Could you check a few things on this model? Use its own coordinates, in mm. A direction names the side the tool comes from. Coordinates: 2 decimals unless noted, no trailing zeros. Order: outer loops, then holes, each group sorted by start corner. A loop starts at its lowest first (then second) coordinate and runs counter-clockwise, first axis right, second up.
```python
from build123d import *

# Parameters (mm, degrees)
ESQUISSE1_W                                   = 30
ESQUISSE1_H                                   = 30
ESQUISSE1_R                                   = 12.5
BOSS_EXTRU_1_DEPTH                            = 6
ESQUISSE3_R                                   = 13
ENL_V_MAT_EXTRU_1_DEPTH                       = 5
TROU_POUR_TARAUDAGE_POUR_TROU_TARAUD_M3_D     = 2.5
TROU_POUR_TARAUDAGE_POUR_TROU_TARAUD_M3_DEPTH = 6
TROU_POUR_TARAUDAGE_POUR_TROU_TARAUD_M3_TIP   = 0.751075774
TROU_POUR_TARAUDAGE_POUR_TROU_TARAUD_2_D      = 2.5
TROU_POUR_TARAUDAGE_POUR_TROU_TARAUD_2_DEPTH  = 6
TROU_POUR_TARAUDAGE_POUR_TROU_TARAUD_2_TIP    = 0.751075774


with BuildPart() as part:
    # Esquisse1 → Boss.-Extru.1 (new body)
    with BuildSketch(Plane.XY):
        with Locations((15, 15)):
            Rectangle(ESQUISSE1_W, ESQUISSE1_H)
        with Locations((15, 15)):
            Circle(ESQUISSE1_R, mode=Mode.SUBTRACT)
    extrude(amount=BOSS_EXTRU_1_DEPTH)

    # Esquisse3 → Enlèv. mat.-Extru.1 (cut)
    with BuildSketch(Plane.XY.offset(6)):
        with Locations((15, 15)):
            Circle(ESQUISSE3_R)
    extrude(amount=-ENL_V_MAT_EXTRU_1_DEPTH, mode=Mode.SUBTRACT)

    # Trou pour taraudage pour trou taraud_ M3
    with Locations(Plane(origin=(0, 30, 0), x_dir=(1, 0, 0), z_dir=(0, 1, 0))):
        with Locations((2, -3), (28, -3)):
            Hole(TROU_POUR_TARAUDAGE_POUR_TROU_TARAUD_M3_D / 2, depth=TROU_POUR_TARAUDAGE_POUR_TROU_TARAUD_M3_DEPTH)
            with Locations((0, 0, -(TROU_POUR_TARAUDAGE_POUR_TROU_TARAUD_M3_DEPTH + TROU_POUR_TARAUDAGE_POUR_TROU_TARAUD_M3_TIP / 2))):  # 118° drill point
                Cone(0, TROU_POUR_TARAUDAGE_POUR_TROU_TARAUD_M3_D / 2, TROU_POUR_TARAUDAGE_POUR_TROU_TARAUD_M3_TIP, mode=Mode.SUBTRACT)

    # Trou pour taraudage pour trou taraud 2
    with Locations(Plane(origin=(0, 0, 0), x_dir=(-1, 0, 0), z_dir=(0, -1, 0))):
        with Locations((-2, -3), (-28, -3)):
            Hole(TROU_POUR_TARAUDAGE_POUR_TROU_TARAUD_2_D / 2, depth=TROU_POUR_TARAUDAGE_POUR_TROU_TARAUD_2_DEPTH)
            with Locations((0, 0, -(TROU_POUR_TARAUDAGE_POUR_TROU_TARAUD_2_DEPTH + TROU_POUR_TARAUDAGE_POUR_TROU_TARAUD_2_TIP / 2))):  # 118° drill point
                Cone(0, TROU_POUR_TARAUDAGE_POUR_TROU_TARAUD_2_D / 2, TROU_POUR_TARAUDAGE_POUR_TROU_TARAUD_2_TIP, mode=Mode.SUBTRACT)


solid = part.part
```
Item 1: Which directions (+Z, -Z, +X, -X, +Y, -Y) give clear straight access to the entire face, cutting with the end or side of a thin tool? Please do faces 1 (the face through (1, 15, 6)), 2 (the face through (29.155, 3.042, 3.479)), 3 (the face through (27.4, 18.9, 3.5)), 4 (the face through (26.845, 26.958, 3.479)).
Item 2: Suppose I cut it at A-A (x = 15). List the corners of the cut face in (y, z) for me, and give its area (3 significant figures).
Item 3: For pin 1 Ø3 at (x, z) = (2, 3) entering from -Y; pin 2 Ø1.5 at (x, z) = (28, 3) entering from -Y; pin 3 Ø2 at (x, z) = (2, 3) entering from -Y, each with a flat end and sliding along its axis, tell me the tip position at first contact or that it passes through.
Item 4: Suppose I cut it at C-C (z = 1.4). List the corners of the cut face in (x, y) for me.
Item 5: I need wall thicknesses on line 1 (Y direction, x = 14.75, z = 0.9); line 2 (Z direction, x = 2, y = 1.5); line 3 (X direction, y = 15.25, z = 4.9). Which ranges of each line are inside material? Lowest first, please.
Item 6: Thinking about a two-plate mould opening in Y: for faces 5 (the face through (27.8, 6.62, 3.08)), 6 (the face through (3.19, 3.04, 2.62)), 7 (the face through (8.2, 25.7, 1)), which applies, +Y half, -Y half, draft (parallel to the pull), parting line (faces both ways), or undercut?
Geometry results:
1. face 1: +Z, +X, -X, +Y, -Y
1. face 2: -Y
1. face 3: +Z
1. face 4: +Y
2. outline: (0, 0) - (2.5, 0) - (2.5, 1) - (2, 1) - (2, 6) - (0, 6) - close; (27.5, 0) - (30, 0) - (30, 6) - (28, 6) - (28, 1) - (27.5, 1) - close
2. area: 25.0 mm2
3. pin 1: stops at y = 0
3. pin 2: stops at y = 6.3
3. pin 3: stops at y = 6.15
4. outline: (0, 0) - (30, 0) - (30, 30) - (0, 30) - close; hole circle Ø26 at (15, 15)
5. line 1: y = 0 to 2.5, 27.5 to 30
5. line 2: z = 0 to 1.75, 4.25 to 6
5. line 3: x = 0 to 2, 28 to 30
6. face 5: -Y half
6. face 6: draft
6. face 7: undercut
